The figure shows three views and two pictorial views of one solid part (mm, origin at its lowest corner). Answer the questions. Round coordinates to 2 decimals unless told otherwise and drop trailing zeros. Order: outer loops, then holes, each group sorted by start corner. A loop starts at its lowest first (then second) coordinate and runs counter-clockwise, first axis right, second up. Notation, with made-up numbers: (-38, -9) - (15, -9) arc R31 ccw to (15, 28) - close; hole circle Ø6 at (19, 76.5). An arc over 180 degrees is marked (long way). One line per item, written item: value. Start each with the question number.
1. Flat-ended cylindrical pins translate along their axes: P1, Ø2, axis at x = 96, z = 117, coming from the +Y side; P2, Ø0.5, axis at x = 72.5, y = 4, coming from the -Z side; P3, Ø0.5, axis at x = 72.5, y = 4, coming from the +Z side. Find the tip coordinate at first contact, or state that the pin passes through.
2. Section B-B, the plane z = 117 is taken. Give the vertices of the cut face in (x, y) (1 decimal).
3. Straight lines are drawn through the part: line 1 (Y direction, x = 51.5, z = 111); line 2 (X direction, y = 3.05, z = 63); line 3 (Z direction, x = 74.5, y = 4.2) (1 decimal). For each, find the intervals that lie inside material, in ascending order.
4. For a pull along X with two mould halves and no side action, classify the marked faces 1 and 2 as released by +X, released by -X, zero draft, split by the parting line, or undercut.
5. Section C-C, the plane x = 60.5 is taken. Give the vertices of the cut face in (y, z).
6. Section D-D, the plane x = 132 is taken. Give the vertices of the cut face in (y, z) (1 decimal).
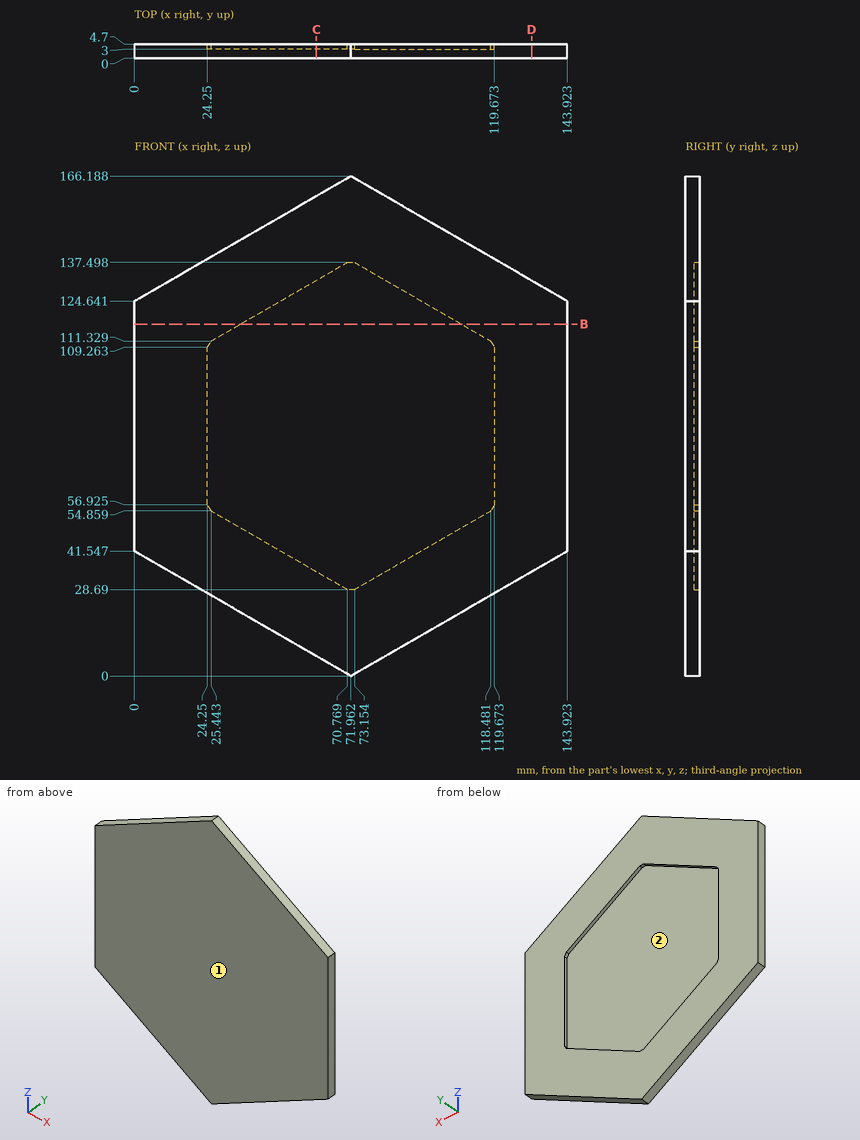
Answer list:
1. P1: stops at y = 3
1. P2: stops at z = 0.17
1. P3: stops at z = 166.02
2. outline: (0, 0) - (143.9, 0) - (143.9, 4.7) - (108.7, 4.7) - (108.7, 3) - (35.3, 3) - (35.3, 4.7) - (0, 4.7) - close
3. line 1: y = 0 to 3
3. line 2: x = 0 to 24.25, 119.67 to 143.92
3. line 3: z = 1.5 to 29.5, 136.7 to 164.7
4. face 1: zero draft
4. face 2: undercut
5. outline: (0, 6.62) - (4.7, 6.62) - (4.7, 34.62) - (3, 34.62) - (3, 131.57) - (4.7, 131.57) - (4.7, 159.57) - (0, 159.57) - close
6. outline: (0, 34.7) - (4.7, 34.7) - (4.7, 131.5) - (0, 131.5) - close
